The model under review builds one solid part; all positions refer to its coordinate system, in mm. A direction names the side the tool comes from. Give positions to 0.01 mm unless a question says otherwise; leave off trailing zeros. Loops run counter-clockwise (first coordinate to the right, second up) from the corner with the lowest first, then second, coordinate; pieces in that order, holes last. Notation, with made-up numbers: (52.5, -31.5) - (66.5, -31.5) arc R8 cw to (66.5, -20.5) - close; hole circle Ø7 at (27, 6). An arc over 180 degrees is marked (long way). Return JSON: item names as keys, results as strings. Group by question number.
from build123d import *

# Parameters (mm, degrees)
SKICA1_W        = 110
SKICA1_H        = 150
SKICA1_W_2      = 90
SKICA1_H_2      = 130
VYSUNOUT1_DEPTH = 8
SKICA2_W        = 90
SKICA2_H        = 130
VYSUNOUT2_DEPTH = 1


with BuildPart() as part:
    # Skica1 → Vysunout1 (new body)
    with BuildSketch(Plane(origin=(0, 0, 0), x_dir=(1, 0, 0), z_dir=(0, 1, 0))):
        Rectangle(SKICA1_W, SKICA1_H)
        Rectangle(SKICA1_W_2, SKICA1_H_2, mode=Mode.SUBTRACT)
    extrude(amount=VYSUNOUT1_DEPTH)

    # Skica2 → Vysunout2 (add)
    with BuildSketch(Plane.XZ):
        Rectangle(SKICA2_W, SKICA2_H)
    extrude(amount=-VYSUNOUT2_DEPTH)


solid = part.part
Item 1: For P1, Ø1.5, axis at x = -13.5, z = -51, coming from the -Y side; P2, Ø3, axis at x = -35.5, z = -7, coming from the +Y side, all flat-tipped, find the tip position at first contact; note any pin that passes through.
Item 2: Tool access review of faces 1 (the face through (-1, 4, -65)), 2 (the face through (55, 4, 1)): name each direction out of +Z, -Z, +X, -X, +Y, -Y from which nothing blocks a thin tool from reaching the whole face with its end or side.
Item 3: Take a section at A-A (x = -6.5). State the section outline as (y, z) points.
Item 4: Mouldability with a two-part tool opening along Z and no side actions: class faces 3 (the face through (-1, 0, 1)), 4 (the face through (-1, 4, 75)), 5 (the face through (-1, 4, 65)) as +Z half, -Z half, draft (parallel to the pull), parting line (faces both ways), or undercut.
Item 5: For L1, parallel to X at y = 2.5, z = -48; L2, parallel to Z at x = 42.5, y = 2.75; L3, parallel to Y at x = 23, z = 18, list the stretches that pass through material, from the lowest coordinate up. Write a range as from..to.
Item 6: Take a section at B-B (y = 6.5). State the section outline as (x, z) points, then the cut area to 3 significant figures.
Item 7: Take a section at C-C (z = 43). State the section outline as (x, y) points.
Check sheet entries:
{
 "1": {"P1": "stops at y = 0", "P2": "stops at y = 1"},
 "2": {"face 1": "+Y", "face 2": "+Z, -Z, +X, +Y, -Y"},
 "3": {"outline": "(0, -75) - (8, -75) - (8, -65) - (1, -65) - (1, 65) - (8, 65) - (8, 75) - (0, 75) - close"},
 "4": {"face 3": "draft", "face 4": "+Z half", "face 5": "undercut"},
 "5": {"L1": "x = -55..-45, 45..55", "L2": "z = -75..-65, 65..75", "L3": "y = 0..1"},
 "6": {"outline": "(-55, -75) - (55, -75) - (55, 75) - (-55, 75) - close; hole (-45, -65) - (45, -65) - (45, 65) - (-45, 65) - close", "area": "4,800 mm^2"},
 "7": {"outline": "(-55, 0) - (55, 0) - (55, 8) - (45, 8) - (45, 1) - (-45, 1) - (-45, 8) - (-55, 8) - close"}
}
